Geometry: see drawing. Coordinates: mm, zero at the bounding-box minimum. Round coordinates to 2 decimals unless told otherwise and drop trailing zeros. Order: outer loops, then holes, each group sorted by start corner. A loop starts at its lowest first (then second) coordinate and runs counter-clockwise, first axis right, second up. Notation, with made-up numbers: (80, -9.5) -> (114, -9.5) arc R32 ccw to (114, 18.5) -> close; hole circle Ø11 at (-32, -22). An arc over 180 degrees is marked (long way). One line per item, written item: value. Start each with the question number.
1) Ray query, L1, parallel to Z at x = 4.25, y = 12; L2, parallel to Z at x = 3.75, y = 7.5; L3, parallel to X at y = 5.5, z = 3. Return the intervals inside material, ascending.
2) Section B-B (x = 6.5). Return the cut outline in (y, z).
3) Section A-A (z = 2.75). Return the cut outline in (x, y).
4) Mould query, pull axis Z, two halves, no side actions, for the marked faces 1, 2 and 3. Classes: pulls with the +Z half, pulls with the -Z half, needs draft (parallel to the pull), parting line crosses it, or undercut.
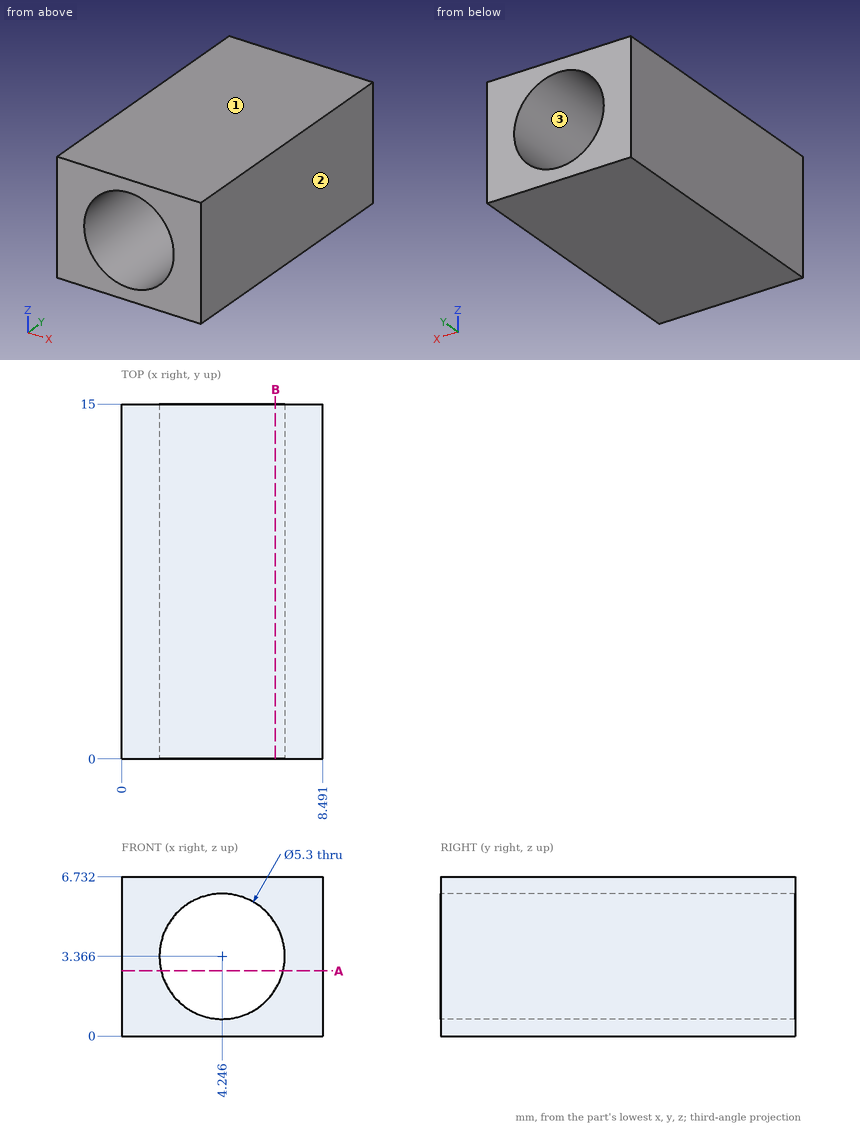
Findings:
1. L1: 0 to 0.72, 6.02 to 6.73
1. L2: 0 to 0.76, 5.97 to 6.73
1. L3: 0 to 1.62, 6.87 to 8.49
2. outline: (0, 0) -> (15, 0) -> (15, 1.97) -> (0, 1.97) -> close; (0, 4.76) -> (15, 4.76) -> (15, 6.73) -> (0, 6.73) -> close
3. outline: (0, 0) -> (1.67, 0) -> (1.67, 15) -> (0, 15) -> close; (6.82, 0) -> (8.49, 0) -> (8.49, 15) -> (6.82, 15) -> close
4. face 1: pulls with the +Z half
4. face 2: needs draft
4. face 3: undercut
